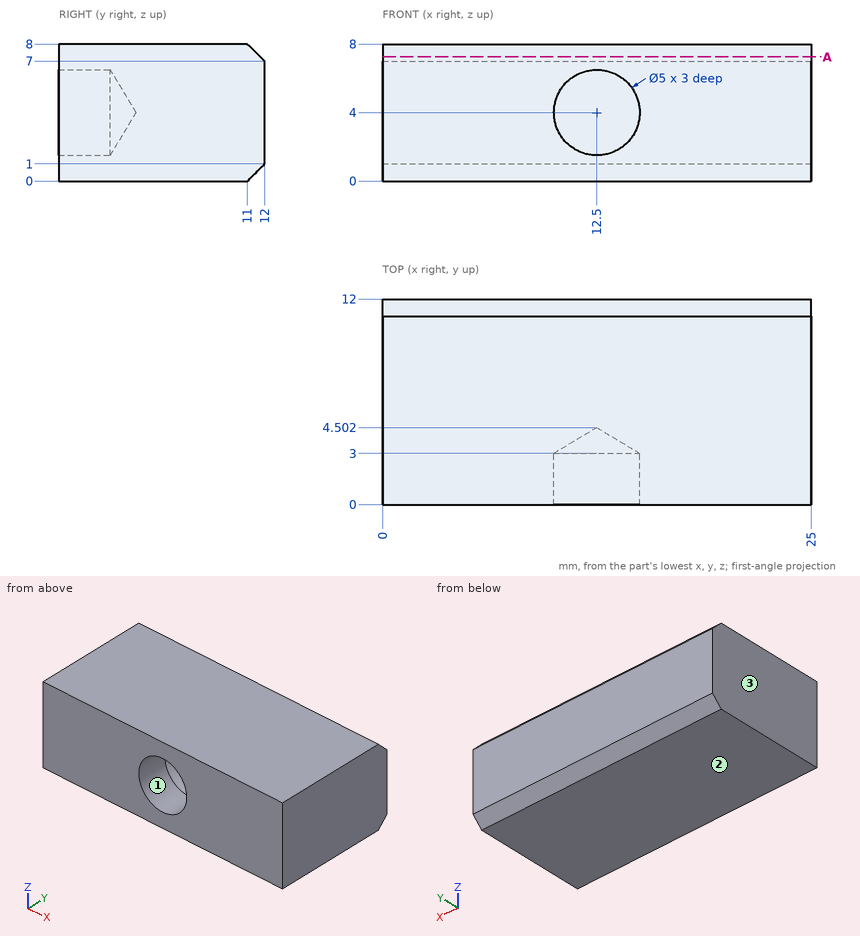
Job drawing, mm, ordinate dimensions from the low corner. One solid piece. Give positions to 0.01 mm unless a question says otherwise; leave off trailing zeros. Loops run counter-clockwise (first coordinate to the right, second up) from the corner with the lowest first, then second, coordinate; pieces in that order, holes last. Notation, with made-up numbers: M 6,58.5 L 61,58.5 A22 cw 61,76.5 Z; hole C 5,-17.5 d8. An arc over 180 degrees is marked long. Use one line per item in the form item = value.
Item 1: Slice it at A-A on z = 7.25. List the corners of the cut face in (x, y).
Filled in:
outline = M 0,0 L 25,0 L 25,11.75 L 0,11.75 Z
Item 2: Drill centre lines: L1, parallel to X at y = 1.3, z = 4; L2, parallel to Z at x = 12.5, y = 2.3; L3, parallel to Z at x = 12, y = 3.75. Where is each one in solid material? Low to high.
Filled in:
L1 = 0 to 10, 15 to 25
L2 = 0 to 1.5, 6.5 to 8
L3 = 0 to 2.85, 5.15 to 8
Item 3: Two-plate mould, pull along X, no slides. Class the marked faces 1, 2 and 3: released by +X, released by -X, zero draft, split by the parting line, or undercut.
Filled in:
face_1 = undercut
face_2 = zero draft
face_3 = released by -X
